Geometry check sheet. Reference: the model listing, model coordinates, mm. Face numbers are marked on the shaded views. A direction names the side the tool comes from. Round coordinates to 2 decimals unless told otherwise and drop trailing zeros. Order: outer loops, then holes, each group sorted by start corner. A loop starts at its lowest first (then second) coordinate and runs counter-clockwise, first axis right, second up.
(1) Cross-section at C-C on z = 22. Enter the section's corners in (x, y).
(2) Thickness scan on L1, parallel to Y at x = 0, z = 13; L2, parallel to Y at x = -14.5, z = 37.5; L3, parallel to X at y = -5, z = 40.5. Record the ranges inside material, lowest first.
(3) Cross-section at D-D on y = -17. Enter the section's corners in (x, z).
(4) Set-up check for the marked faces 1 and 2: record each of +Z, -Z, +X, -X, +Y, -Y from which the full face is reachable in a straight line by a thin tool's end or side.
(5) Draft check along X on the marked faces 3, 4 and 5. Enter one of: pulls with the +X half, pulls with the -X half, needs draft (parallel to the pull), parting line crosses it, or undercut.
(6) Gauge pin test, flat end, axial feed: P1, Ø5, axis at x = -3, y = -3.5, coming from the +Z side. Record the tip position at first contact, or that the pin passes through.
(7) Cross-section at A-A on x = 0. Enter the section's corners in (y, z), and give its area (3 significant figures).
from build123d import *

# Parameters (mm, degrees)
F0_R     = 11.5
F0_R_2   = 9.5
F1_DEPTH = 60
F0_W     = 44
F0_H     = 44
F0_W_2   = 40
F0_H_2   = 40
F2_DEPTH = 60
F3_DEPTH = 2


with BuildPart() as f1:
    # F0 (on Top) → F1 (new body)
    with BuildSketch(Plane.XY):
        Circle(F0_R)
        Circle(F0_R_2, mode=Mode.SUBTRACT)
    extrude(amount=F1_DEPTH)



with BuildPart() as f2:
    # F0 (on Top) → F2 (new body)
    with BuildSketch(Plane.XY):
        Rectangle(F0_W, F0_H)
        Rectangle(F0_W_2, F0_H_2, mode=Mode.SUBTRACT)
    extrude(amount=F2_DEPTH)


with BuildPart() as f1_1:
    add(f1.part)

    add(f2.part)  # F3 merges F2
    # F0 (on Top) → F3 (join)
    with BuildSketch(Plane.XY):
        Rectangle(F0_W_2, F0_H_2)
        Circle(F0_R, mode=Mode.SUBTRACT)
    extrude(amount=F3_DEPTH)


solid = f1_1.part
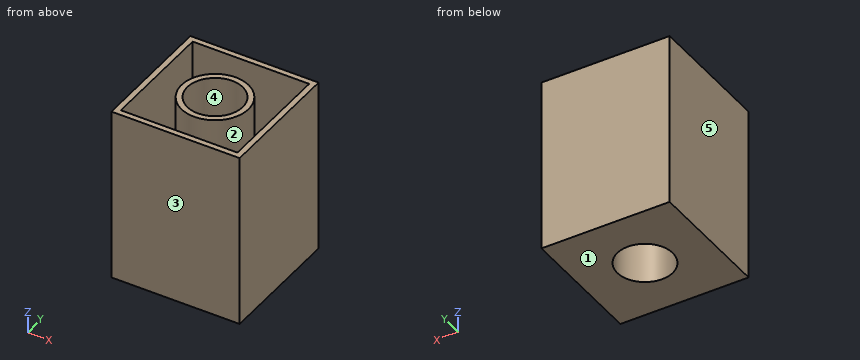
Found:
1. outline: (-22, -22) - (22, -22) - (22, 22) - (-22, 22) - close; circle Ø23 at (0, 0); hole (-20, -20) - (20, -20) - (20, 20) - (-20, 20) - close; hole circle Ø19 at (0, 0)
2. L1: y = -22 to -20, -11.5 to -9.5, 9.5 to 11.5, 20 to 22
2. L2: y = -22 to -20, 20 to 22
2. L3: x = -22 to -20, -10.36 to -8.08, 8.08 to 10.36, 20 to 22
3. outline: (-22, 0) - (22, 0) - (22, 60) - (20, 60) - (20, 2) - (-20, 2) - (-20, 60) - (-22, 60) - close
4. face 1: -Z, +X, -X, +Y, -Y
4. face 2: +Z
5. face 3: needs draft
5. face 4: undercut
5. face 5: pulls with the -X half
6. P1: passes through
7. outline: (-22, 0) - (-9.5, 0) - (-9.5, 60) - (-11.5, 60) - (-11.5, 2) - (-20, 2) - (-20, 60) - (-22, 60) - close; (9.5, 0) - (22, 0) - (22, 60) - (20, 60) - (20, 2) - (11.5, 2) - (11.5, 60) - (9.5, 60) - close
7. area: 514 mm2
